Part print with two shaded views. Sizes in mm from the minimum x, y, z corner. Give positions to 0.01 mm unless a question says otherwise; leave off trailing zeros. Write each loop counter-clockwise with the first axis right and the second up, starting at its lowest first coordinate (ties: lowest second). Pieces come first, ordered by that corner, then holes. Notation, with made-up numbers: (15, 64.5) - (49, 64.5) arc R14 cw to (49, 82.5) - close; hole circle Ø5 at (9.5, 44). An arc over 180 degrees is marked (long way). Answer as a JSON object with one key per item and string values. Group by question number.
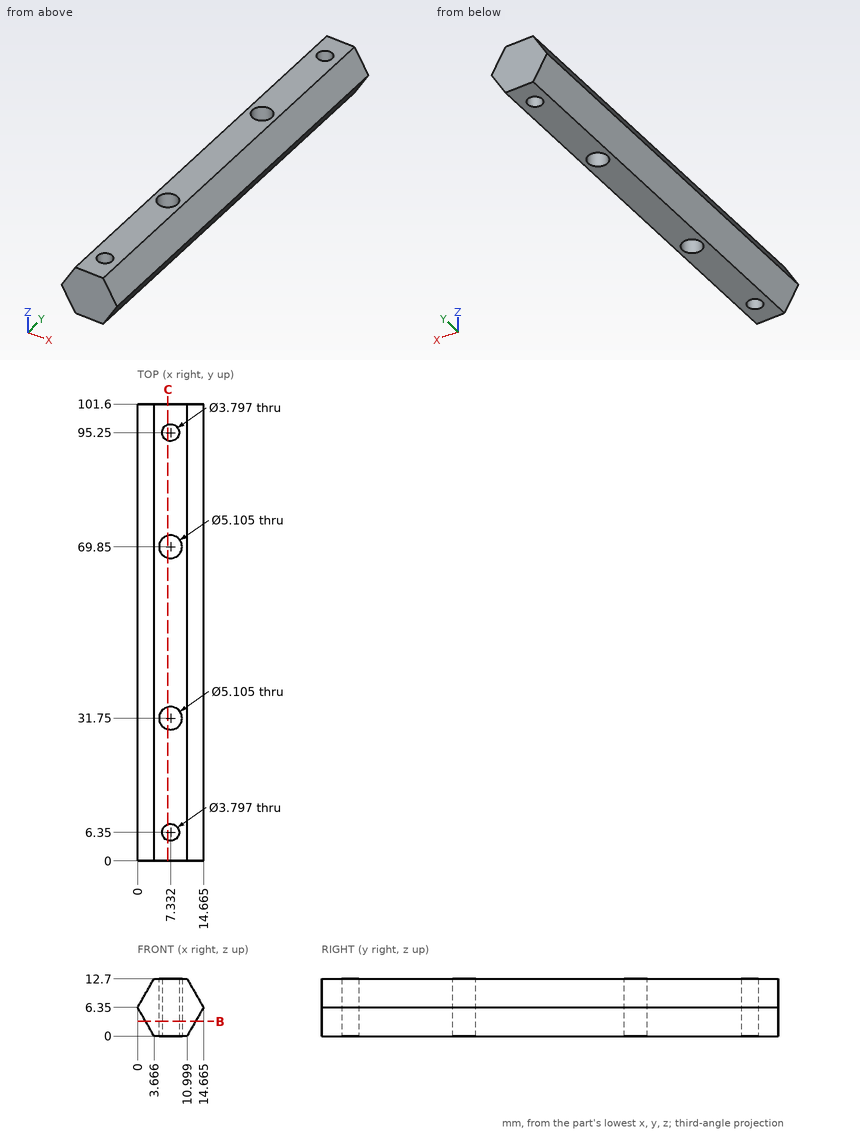
1) Saw through at C-C (x = 6.75). List the corners of the cut face in (y, z) (1 decimal).
2) Drill centre lines: line 1 along Y through (x, z) = (8.5, 1) (1 decimal); line 2 along Y through (x, z) = (9, 10.5) (1 decimal); line 3 along Z through (x, y) = (11, 14) (1 decimal). Where is each one in solid material? Low to high. Write a range as from..to.
3) Drop flat-ended pins along their axis: P1, Ø5, axis at x = 10.5, y = 15, coming from the -Z side; P2, Ø3.5, axis at x = 7.33, y = 6.35, coming from the +Z side; P3, Ø6, axis at y = 19, z = 3.5, coming from the -X side. Give the stop position or say it passes through.
4) Saw through at B-B (z = 3.25). State how many separate pieces and enclosed holes the cut face has, and give its area (3 significant figures).
Checks:
{
 "1": {"outline": "(0, 0) - (4.5, 0) - (4.5, 12.7) - (0, 12.7) - close; (8.2, 0) - (29.3, 0) - (29.3, 12.7) - (8.2, 12.7) - close; (34.2, 0) - (67.4, 0) - (67.4, 12.7) - (34.2, 12.7) - close; (72.3, 0) - (93.4, 0) - (93.4, 12.7) - (72.3, 12.7) - close; (97.1, 0) - (101.6, 0) - (101.6, 12.7) - (97.1, 12.7) - close"},
 "2": {"line 1": "0..4.9, 7.8..29.5, 34..67.6, 72.1..93.8, 96.7..101.6", "line 2": "0..5.4, 7.3..29.8, 33.7..67.9, 71.8..94.3, 96.2..101.6", "line 3": "0..12.7"},
 "3": {"P1": "z = 0", "P2": "through", "P3": "x = 0"},
 "4": {"separate pieces": "1", "enclosed holes": "4", "area": "1,060 mm2"}
}
